Geometry check sheet. Reference: the model listing, model coordinates, mm. Face numbers are marked on the shaded views. A direction names the side the tool comes from. Give positions to 0.01 mm unless a question says otherwise; leave off trailing zeros. Order: outer loops, then holes, each group sorted by start corner. A loop starts at its lowest first (then second) coordinate and runs counter-clockwise, first axis right, second up. Notation, with made-up numbers: M 50.25,10 L 87.25,10 A17 ccw 87.25,14 Z; hole C -35,-29 d2. An arc over 180 degrees is marked long. Answer as a JSON object with one key per item and string values. Group by question number.
from build123d import *

# Parameters (mm, degrees)
F0_W     = 152.4
F0_H     = 101.6
F1_DEPTH = 38.1
F2_W     = 12.7
F2_H     = 101.6
F3_DEPTH = 25.4
F4_W     = 152.4
F4_H     = 32.6725877821
F5_DEPTH = 38.1
F6_W     = 12.7
F6_H     = 34.8848986059
F7_DEPTH = 76.201


with BuildPart() as f1:
    # F0 (on Top) → F1 (new body, symmetric)
    with BuildSketch(Plane.XY):
        Rectangle(F0_W, F0_H)
    extrude(amount=F1_DEPTH, both=True)

    # F2 (on face) → F3 (cut)
    with BuildSketch(Plane.XY.offset(38.1)):
        with Locations((44.45, 0)):
            Rectangle(F2_W, F2_H)
    extrude(amount=-F3_DEPTH, mode=Mode.SUBTRACT)

    # F4 (on face) → F5 (cut)
    with BuildSketch(Plane.XY.offset(38.1)):
        with Locations((0, 0.421192497)):
            Rectangle(F4_W, F4_H)
    extrude(amount=-F5_DEPTH, mode=Mode.SUBTRACT)

    # F6 (on face) → F7 (intersect, through all)
    with BuildSketch(Plane.XY.offset(38.1)):
        Polygon((38.1, -15.9151013941), (38.1, -50.8), (76.2, -50.8), (76.2, 50.8), (50.8, 50.8), (25.4, 50.8), (25.4, -15.9151013941), align=None)
        with Locations((31.75, -33.357550697)):
            Rectangle(F6_W, F6_H)
    extrude(amount=-F7_DEPTH, mode=Mode.INTERSECT)


solid = f1.part
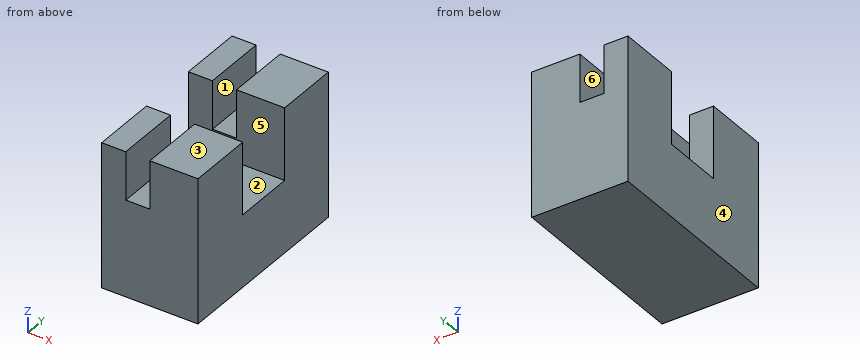
1. Cross-section at C-C (z = 3.5). Record the cut outline in (x, y), and give its area (3 significant figures).
2. Thickness scan on line 1 along X through (y, z) = (-37, 24); line 2 along Y through (x, z) = (33.5, 4.5); line 3 along Z through (x, y) = (64, -8). Record the ranges inside material, lowest first. Write a range as [from, to].
3. Cross-section at D-D (y = -20). Record the cut outline in (x, z), and give its area (3 significant figures).
4. Release check for a two-part mould opening along X. For the marked faces 4, 5 and 6 record: released by +X, released by -X, zero draft, split by the parting line, or undercut.
5. Access from +Z, -Z, +X, -X, +Y, -Y to the whole of each face (thin tool, end or side, straight path). Record for the marked faces 1, 2 and 3.
6. Cross-section at B-B (x = 45). Record the cut outline in (y, z).
7. Cross-section at A-A (z = 16). Record the cut outline in (x, y).
8. Depth check by flat-ended pin: pin 1 (16.5 mm diameter, centred on x = 48.5, y = 2.5, fed in from +Z). Enter the tip coordinate at first touch or a pass-through.
Report:
{
 "1": {"outline": "M 25.4,-50.8 L 76.2,-50.8 L 76.2,-15.92 L 25.4,-15.92 Z; M 25.4,16.76 L 76.2,16.76 L 76.2,50.8 L 25.4,50.8 Z", "area": "3,500 mm2"},
 "2": {"line 1": "x = [25.4, 38.1], [50.8, 76.2]", "line 2": "y = [-50.8, -15.92], [16.76, 50.8]", "line 3": "z = [-38.1, 0]"},
 "3": {"outline": "M 25.4,-38.1 L 76.2,-38.1 L 76.2,38.1 L 50.8,38.1 L 50.8,12.7 L 38.1,12.7 L 38.1,38.1 L 25.4,38.1 Z", "area": "3,550 mm2"},
 "4": {"face 4": "released by -X", "face 5": "zero draft", "face 6": "undercut"},
 "5": {"face 1": "+Z, +Y, -Y", "face 2": "+Z, +X, -X", "face 3": "+Z, +X, -X, +Y, -Y"},
 "6": {"outline": "M -50.8,-38.1 L 50.8,-38.1 L 50.8,12.7 L 16.76,12.7 L 16.76,0 L -15.92,0 L -15.92,12.7 L -50.8,12.7 Z"},
 "7": {"outline": "M 25.4,-50.8 L 38.1,-50.8 L 38.1,-15.92 L 25.4,-15.92 Z; M 25.4,16.76 L 38.1,16.76 L 38.1,50.8 L 25.4,50.8 Z; M 50.8,-50.8 L 76.2,-50.8 L 76.2,-15.92 L 50.8,-15.92 Z; M 50.8,16.76 L 76.2,16.76 L 76.2,50.8 L 50.8,50.8 Z"},
 "8": {"pin 1": "stops at z = 0"}
}
